Can you work these out from the model? Positions are in its coordinate system, mm. A direction names the side the tool comes from. Round coordinates to 2 decimals unless told otherwise and drop trailing zeros. Write each loop counter-clockwise with the first axis right and the second up, starting at its lowest first coordinate (ties: lowest second). Pieces come first, ordered by that corner, then holes.
Q1. We'd pull the mould along Z, two halves only. Please class faces 4 (the flat face through (5.4, 1.1, -1.5)), 5 (the flat face through (0, 0, 2)), 6 (the cylindrical face through (27.99, -0.9, 2.86)): +Z half, -Z half, draft (parallel to the pull), parting line (faces both ways), or undercut.
Q2. If we section it at C-C (z = 0): Please give me the cut outline in (x, y) (3 decimals), plus the area to 3 significant figures.
Q3. If we section it at D-D (z = -2.5): Give the number of separate pieces and of enclosed holes in the cut face, plus the area to 3 significant figures.
Q4. I'm going to push flat-ended pins straight in: pin 1 Ø1.6 at (x, y) = (4, -1) entering from -Z; pin 2 Ø2 at (y, z) = (-1, 1) entering from -X; pin 3 Ø1.5 at (y, z) = (0.5, 0) entering from -X; pin 4 Ø1 at (x, z) = (4, 1.5) entering from +Y. Where does each tip first touch, or does it pass through?
Q5. For faces 1 (the flat face through (5.4, 1.1, 1.5)), 2 (the flat face through (26, 2, -1.3)), 3 (the cylindrical face through (16, -3, 0)), which set-ups out of +Z, -Z, +X, -X, +Y, -Y let a thin tool reach every point of the face, with its end or its side?
Q6. Please list where these lines run through material, in increasing order: line 1 along X through (y, z) = (-0.75, 1); line 2 along Y through (x, z) = (4, 2.45); line 3 along Z through (x, y) = (7, 1).
Q7. If we section it at B-B (y = 0): Please give me the cut outline in (x, z) (3 decimals).
Q8. If we section it at A-A (x = 4): Please give me the cut outline in (y, z), plus the area to 3 significant figures.
from build123d import *

# Parameters (mm, degrees)
CUT_EXTRUDE1_DEPTH      = 31.298514815
CUT_EXTRUDE1_DEPTH_BACK = 31.298514815
SKETCH2_W               = 9
SKETCH2_H               = 3
CUT_EXTRUDE2_DEPTH      = 31.298514815
CUT_EXTRUDE2_DEPTH_BACK = 31.298514815
SKETCH3_R               = 1.5


with BuildPart() as part:
    # Sketch1 → Revolve1 (revolve)
    with BuildSketch(Plane.XY, mode=Mode.PRIVATE) as revolve1_sk:
        Polygon((30, 0), (30, 2), (29, 3), (27, 3), (27, 2.125), (26, 2.125), (26, 3), (0, 3), (0, 0), align=None)
    revolve(revolve1_sk.sketch.rotate(Axis((0, 0, 0), (1, 0, 0)), 90), axis=Axis((0, 0, 0), (1, 0, 0)))

    # Sketch2 → Cut-Extrude1 (cut, two sides: drawn at the far end of the back side and taken through both)
    with BuildSketch(Plane(origin=(0, 0, 0), x_dir=(1, 0, 0), z_dir=(0, 1, 0)).offset(-CUT_EXTRUDE1_DEPTH_BACK)):
        with Locations((4.5, 0)):
            Rectangle(SKETCH2_W, SKETCH2_H)
    extrude(amount=CUT_EXTRUDE1_DEPTH + CUT_EXTRUDE1_DEPTH_BACK, mode=Mode.SUBTRACT)

    # Sketch3 → Cut-Extrude2 (cut, two sides: drawn at the far end of the back side and taken through both)
    with BuildSketch(Plane.XY.offset(-CUT_EXTRUDE2_DEPTH_BACK)):
        with Locations((4, 0)):
            Circle(SKETCH3_R)
    extrude(amount=CUT_EXTRUDE2_DEPTH + CUT_EXTRUDE2_DEPTH_BACK, mode=Mode.SUBTRACT)


solid = part.part
A:
1. face 4: undercut
1. face 5: draft
1. face 6: parting line
2. outline: (9, -3) - (26, -3) - (26, -2.125) - (27, -2.125) - (27, -3) - (29, -3) - (30, -2) - (30, 2) - (29, 3) - (27, 3) - (27, 2.125) - (26, 2.125) - (26, 3) - (9, 3) - close
2. area: 123 mm2
3. separate pieces: 2
3. enclosed holes: 1
3. area: 86.9 mm2
4. pin 1: stops at z = -2.7
4. pin 2: stops at x = 0
4. pin 3: stops at x = 9
4. pin 4: stops at y = 2.6
5. face 1: -X, +Y, -Y
5. face 2: none
5. face 3: +X, -X
6. line 1: x = 9 to 30
6. line 2: y = -1.73 to -1.5, 1.5 to 1.73
6. line 3: z = -2.83 to -1.5, 1.5 to 2.83
7. outline: (0, -3) - (2.5, -3) - (2.5, -1.5) - (0, -1.5) - close; (0, 1.5) - (2.5, 1.5) - (2.5, 3) - (0, 3) - close; (5.5, -3) - (26, -3) - (26, -2.125) - (27, -2.125) - (27, -3) - (29, -3) - (30, -2) - (30, 2) - (29, 3) - (27, 3) - (27, 2.125) - (26, 2.125) - (26, 3) - (5.5, 3) - (5.5, 1.5) - (9, 1.5) - (9, -1.5) - (5.5, -1.5) - close
8. outline: (-2.6, -1.5) arc R3 ccw to (-1.5, -2.6) - (-1.5, -1.5) - close; (-2.6, 1.5) - (-1.5, 1.5) - (-1.5, 2.6) arc R3 ccw to start; (1.5, -2.6) arc R3 ccw to (2.6, -1.5) - (1.5, -1.5) - close; (1.5, 1.5) - (2.6, 1.5) arc R3 ccw to (1.5, 2.6) - close
8. area: 2.84 mm2
